The listing builds one solid part. Answer for the finished solid, in the listing's coordinates (mm). A direction names the side the tool comes from. Give positions to 0.01 mm unless a question says otherwise; leave off trailing zeros. Loops run counter-clockwise (first coordinate to the right, second up) from the corner with the lowest first, then second, coordinate; pieces in that order, holes last. Notation, with made-up numbers: M -27,23.5 L -11,23.5 A14 ccw -11,33.5 Z; hole C -10.75,9.25 d2. An arc over 180 degrees is marked long. Return JSON: item names as keys, results as strings.
from build123d import *

# Parameters (mm, degrees)
SKETCH1_R                       = 25
BOSS_EXTRUDE1_DEPTH             = 15
CBORE_FOR_M4_SHCS1_AT_2_COUNT   = 2
CBORE_FOR_M4_SHCS1_AT_2_PITCH   = 16
CBORE_FOR_M4_SHCS1_AT_3_COUNT   = 2
CBORE_FOR_M4_SHCS1_AT_3_PITCH   = 22.627416998
CBORE_FOR_M4_SHCS1_AT_4_COUNT   = 2
CBORE_FOR_M4_SHCS1_AT_4_PITCH   = 16
F_10_0MM_DOWEL_HOLE1_D          = 10
F_9_64_0_14063_DIAMETER_HOLE1_D = 3.572002
SKETCH9_W                       = 18
SKETCH9_H                       = 12
CUT_EXTRUDE1_DEPTH              = 2
FILLET2_R                       = 1
CUT_EXTRUDE2_DEPTH              = 39.405728739
FILLET3_START                   = -1
FILLET3_DEPTH                   = 17


with BuildPart() as part:
    # Sketch1 → Boss-Extrude1 (new body)
    with BuildSketch(Plane(origin=(0, 0, 0), x_dir=(1, 0, 0), z_dir=(0, 1, 0))):
        with Locations(Location((0, 0, 0), (0, 0, 270))):
            Circle(SKETCH1_R)
    extrude(amount=BOSS_EXTRUDE1_DEPTH)

    # Sketch4 → CBORE for M4 SHCS1 (revolve, cut)
    with BuildSketch(Plane(origin=(-8, 15, -8), x_dir=(0, 0, 1), z_dir=(1, 0, 0))):
        Polygon((0, 0), (0, 15), (2.25, 15), (2.25, 11), (4, 11), (4, 0.025), (4.025, 0), align=None)
    cbore_for_m4_shcs1 = revolve(axis=Axis((-8, 21.35, -8), (0, -1, 0)), mode=Mode.SUBTRACT)

    # CBORE for M4 SHCS1 at 2: CBORE for M4 SHCS1 ×2
    with Locations(*[(i * CBORE_FOR_M4_SHCS1_AT_2_PITCH, 0, 0) for i in range(1, CBORE_FOR_M4_SHCS1_AT_2_COUNT)]):
        add(cbore_for_m4_shcs1, mode=Mode.SUBTRACT)

    # CBORE for M4 SHCS1 at 3: CBORE for M4 SHCS1 ×2
    with Locations(*[Vector(0.7071067811865476, 0, 0.7071067811865476) * (i * CBORE_FOR_M4_SHCS1_AT_3_PITCH) for i in range(1, CBORE_FOR_M4_SHCS1_AT_3_COUNT)]):
        add(cbore_for_m4_shcs1, mode=Mode.SUBTRACT)

    # CBORE for M4 SHCS1 at 4: CBORE for M4 SHCS1 ×2
    with Locations(*[(0, 0, i * CBORE_FOR_M4_SHCS1_AT_4_PITCH) for i in range(1, CBORE_FOR_M4_SHCS1_AT_4_COUNT)]):
        add(cbore_for_m4_shcs1, mode=Mode.SUBTRACT)

    # Ø10.0mm Dowel Hole1 (through all)
    with Locations(Plane(origin=(0, 15, 0), x_dir=(1, 0, 0), z_dir=(0, 1, 0))):
        with Locations((0, 0)):
            Hole(F_10_0MM_DOWEL_HOLE1_D / 2)

    # 9/64 (0.14063) Diameter Hole1 (through all)
    with Locations(Plane(origin=(0, 15, 0), x_dir=(1, 0, 0), z_dir=(0, 1, 0))):
        with Locations((-20, 0), (20, 0)):
            Hole(F_9_64_0_14063_DIAMETER_HOLE1_D / 2)

    # Sketch9 → Cut-Extrude1 (cut)
    with BuildSketch(Plane(origin=(0, 15, 0), x_dir=(1, 0, 0), z_dir=(0, 1, 0))):
        with Locations((-18.5, 0)):
            Rectangle(SKETCH9_W, SKETCH9_H)
    cut_extrude1 = extrude(amount=-CUT_EXTRUDE1_DEPTH, mode=Mode.SUBTRACT)

    # Mirror1: Cut-Extrude1 across plane
    add(cut_extrude1.mirror(Plane(origin=(0, 0, 0), x_dir=(0, 0, 1), z_dir=(1, 0, 0))), mode=Mode.SUBTRACT)

    # Fillet2
    fillet2_edges = [part.edges().sort_by_distance(p)[0] for p in [
        (-24.269322199, 14, -6),
        (-24.269322199, 14, 6),
        (-11.464101615, 13.9875, 6),
        (-9.5, 13.9875, 4.291900756),
        (-11.464101615, 13.9875, -6),
        (-9.5, 13.9875, -4.291900756),
        (24.269322199, 14, 6),
        (9.5, 13.9875, 4.291900756),
        (9.5, 13.9875, -4.291900756),
        (24.269322199, 14, -6),
        (11.464101615, 13.9875, -6),
        (11.464101615, 13.9875, 6),
    ]]
    fillet(fillet2_edges, radius=FILLET2_R)

    # Sketch10 → Cut-Extrude2 (cut, through all)
    with BuildSketch(Plane(origin=(0, 15, 0), x_dir=(1, 0, 0), z_dir=(0, 1, 0))):
        with BuildLine():
            ThreePointArc((21.354156504, 13), (0, 25), (-21.354156504, 13))
            Line((-21.354156504, 13), (21.354156504, 13))
        make_face()
    extrude(amount=-CUT_EXTRUDE2_DEPTH, mode=Mode.SUBTRACT)

    # Fillet3: read off the stored shape, not the designer's step
    # Fillet3 outline → Fillet3 (cut)
    with BuildSketch(Plane(origin=(0, 0, 0), x_dir=(1, 0, 0), z_dir=(0, 1, 0)).offset(FILLET3_START)):
        with BuildLine():
            Line((21.354156504, 13), (14.696938457, 13))
            ThreePointArc((14.696938457, 13), (21.021493777, 10.745966692), (24.494897428, 5))
            ThreePointArc((24.494897428, 5), (23.270881733, 9.135976324), (21.354156504, 13))
        make_face()
        with BuildLine():
            Line((-14.696938457, 13), (-21.354156504, 13))
            ThreePointArc((-21.354156504, 13), (-23.270881733, 9.135976324), (-24.494897428, 5))
            ThreePointArc((-24.494897428, 5), (-21.021493777, 10.745966692), (-14.696938457, 13))
        make_face()
    extrude(amount=FILLET3_DEPTH, mode=Mode.SUBTRACT)


solid = part.part
(1) Given pin 1 (10 mm diameter, centred on x = 17.5, z = 3, fed in from +Y); pin 2 (0.6 mm diameter, centred on x = -15.5, y = 14.5, fed in from -Z); pin 3 (6 mm diameter, centred on x = 8, z = -8, fed in from +Y); pin 4 (2 mm diameter, centred on x = -19, y = 14, fed in from +Z), each flat-ended and moving along its own axis, determine where each tip first touches the part or whether it passes through.
Values follow:
{"pin 1": "y = 15", "pin 2": "z = -12.99", "pin 3": "y = 4", "pin 4": "z = 17.35"}
(2) The part is cut by section B-B (z = 0). Determine the outline of the cut face in (x, y).
Values follow:
{"outline": "M -25,0 L -21.79,0 L -21.79,13 L -25,13 Z; M -18.21,0 L -5,0 L -5,15 L -9.5,15 L -9.5,13 L -18.21,13 Z; M 5,0 L 18.21,0 L 18.21,13 L 9.5,13 L 9.5,15 L 5,15 Z; M 21.79,0 L 25,0 L 25,13 L 21.79,13 Z"}
(3) Straight lines are drawn through the part: line 1 along Z through (x, y) = (-8, 2); line 2 along X through (y, z) = (11.5, -8); line 3 along X through (y, z) = (10, 4.5). For each, find the intervals that lie inside material, in ascending order.
Values follow:
{"line 1": "-13 to -10.25, -5.75 to 5.75, 10.25 to 23.69", "line 2": "-23.36 to -12, -4 to 4, 12 to 23.36", "line 3": "-24.59 to -9.94, -6.06 to -2.18, 2.18 to 6.06, 9.94 to 24.59"}
(4) The part is cut by section D-D (z = 8). Determine the outline of the cut face in (x, y) (3 decimals), and give its area (3 significant figures).
Values follow:
{"outline": "M -23.685,0 L -10.25,0 L -10.25,4 L -12,4 L -12,14.975 L -12.025,15 L -23.685,15 Z; M -5.75,0 L 5.75,0 L 5.75,4 L 4,4 L 4,14.975 L 3.975,15 L -3.975,15 L -4,14.975 L -4,4 L -5.75,4 Z; M 10.25,0 L 23.685,0 L 23.685,15 L 12.025,15 L 12,14.975 L 12,4 L 10.25,4 Z", "area": "499 mm²"}
(5) Determine the mould class of faces 6 (the cylindrical face through (-23.603, 13.986, -6.237)), 7 (the flat face through (0, 0, 6)), 8 (the flat face through (-6, 4, -10)) for opening direction X: released by +X, released by -X, zero draft, split by the parting line, or undercut.
Values follow:
{"face 6": "released by -X", "face 7": "zero draft", "face 8": "undercut"}
(6) The part is cut by section C-C (y = 9). Determine the outline of the cut face in (x, z), and give its area (3 significant figures).
Values follow:
{"outline": "M -24.49,-5 A10 ccw -14.7,-13 L 14.7,-13 A10 ccw 24.49,-5 A25 ccw long Z; hole C -20,0 d3.57; hole C -8,-8 d8; hole C -8,8 d8; hole C 0,0 d10; hole C 8,-8 d8; hole C 8,8 d8; hole C 20,0 d3.57", "area": "1,280 mm²"}
(7) A tool of negligible diameter and unlimited length cuts with its end or side. For faces 1 (the cylindrical face through (-23.77, 13.99, 6.42)), 2 (the cylindrical face through (-9.52, 2.03, -9.66)), 3 (the flat face through (0, 15, 6)), 4 (the cylindrical face through (23.603, 13.986, -6.237)), 5 (the cylindrical face through (-5.6, 9.6, -11.2)), from which of +Z, -Z, +X, -X, +Y, -Y can it reach the whole face along a straight path? Write none if from no direction.
Values follow:
{"face 1": "-X, +Y", "face 2": "+Y, -Y", "face 3": "+Z, -Z, +X, -X, +Y", "face 4": "+X, +Y", "face 5": "+Y"}
(8) The part is cut by section A-A (x = 0). Determine the outline of the cut face in (y, z), and give its area (3 significant figures).
Values follow:
{"outline": "M 0,-13 L 15,-13 L 15,-5 L 0,-5 Z; M 0,5 L 15,5 L 15,25 L 0,25 Z", "area": "420 mm²"}
